Build history of the part. All positions in model axes, mm. Coordinates: 2 decimals unless noted, no trailing zeros. Loops run counter-clockwise (first coordinate to the right, second up) from the corner with the lowest first, then second, coordinate; pieces in that order, holes last.
Item 1: Cut at A-A (x = 0). List the corners of the cut face in (y, z), and give its area (3 significant figures).
Item 2: Drill centre lines: line 1 along Y through (x, z) = (0, 132); line 2 along X through (y, z) = (1.5, 173); line 3 along Y through (x, z) = (1.75, 93.5). Where is each one in solid material? Low to high.
Item 3: Flat gauge pins, fed straight in: pin 1 (1.9 mm diameter, centred on x = 6.5, z = 22, fed in from -Y); pin 2 (1.9 mm diameter, centred on x = -7, z = 20.5, fed in from +Y); pin 3 (1.4 mm diameter, centred on x = 7, y = 0, fed in from -Z); pin 4 (4 mm diameter, centred on x = 6, y = 5.5, fed in from +Z). Where does each tip first touch, or does it go through?
Item 4: Cut at B-B (z = 285.5). List the corners of the cut face in (x, y).
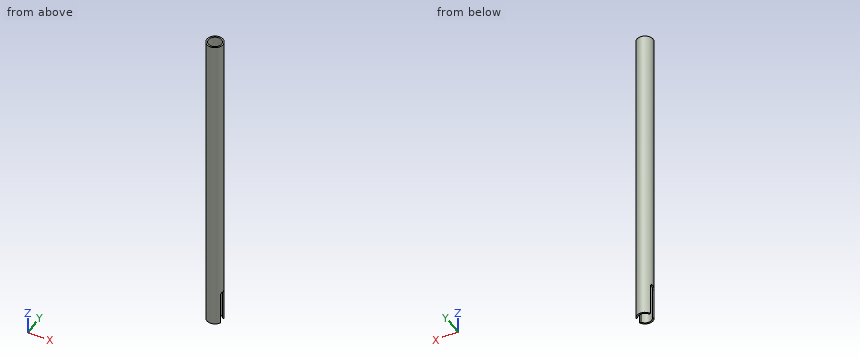
from build123d import *

# Parameters (mm, degrees)
SKETCH1_R               = 8.001
SKETCH1_R_2             = 6.477
BOSS_EXTRUDE1_DEPTH     = 312.42
CUT_EXTRUDE2_DEPTH      = 313.624836509
CUT_EXTRUDE2_DEPTH_BACK = 313.624836509


with BuildPart() as part:
    # Sketch1 → Boss-Extrude1 (new body)
    with BuildSketch(Plane.XY):
        Circle(SKETCH1_R)
        Circle(SKETCH1_R_2, mode=Mode.SUBTRACT)
    extrude(amount=BOSS_EXTRUDE1_DEPTH)

    # Sketch2 → Cut-Extrude2 (cut, two sides: drawn at the far end of the back side and taken through both)
    with BuildSketch(Plane(origin=(0, 0, 0), x_dir=(0, 0, -1), z_dir=(1, 0, 0)).offset(-CUT_EXTRUDE2_DEPTH_BACK)):
        with BuildLine():
            Line((635.239664052, 3.175), (0, 3.175))
            Line((0, 3.175), (-31.75, 3.175))
            ThreePointArc((-31.75, 3.175), (-32.827630735, 2.728630735), (-33.274, 1.651))
            Line((-33.274, 1.651), (-33.274, -1.651))
            ThreePointArc((-33.274, -1.651), (-32.827630735, -2.728630735), (-31.75, -3.175))
            Line((-31.75, -3.175), (0, -3.175))
            Line((0, -3.175), (635.239664052, -3.175))
            Line((635.239664052, -3.175), (1905.718992156, -3.175))
            Line((1905.718992156, -3.175), (1905.718992156, 3.175))
            Line((1905.718992156, 3.175), (635.239664052, 3.175))
        make_face()
    extrude(amount=CUT_EXTRUDE2_DEPTH + CUT_EXTRUDE2_DEPTH_BACK, mode=Mode.SUBTRACT)


solid = part.part
Filled sheet:
1. outline: (-8, 0) - (-6.48, 0) - (-6.48, 312.42) - (-8, 312.42) - close; (6.48, 0) - (8, 0) - (8, 312.42) - (6.48, 312.42) - close
1. area: 952 mm2
2. line 1: y = -8 to -6.48, 6.48 to 8
2. line 2: x = -7.86 to -6.3, 6.3 to 7.86
2. line 3: y = -7.81 to -6.24, 6.24 to 7.81
3. pin 1: stops at y = -5.76
3. pin 2: stops at y = 5.24
3. pin 3: stops at z = 33.27
3. pin 4: stops at z = 312.42
4. outline: circle Ø16 at (0, 0); hole circle Ø12.95 at (0, 0)
